Input: part model. Units: mm. Frame: model coordinates. A direction names the side the tool comes from. Round coordinates to 2 decimals unless told otherwise and drop trailing zeros. Order: outer loops, then holes, each group sorted by start corner. A loop starts at its lowest first (then second) coordinate and runs counter-clockwise, first axis right, second up.
Item 1: First-contact query: pin 1 (11 mm diameter, centred on x = 0, z = 5, fed in from -Y). Flat tip, straight axial feed; report the tip coordinate or a pass-through.
Item 2: Cut plane C-C on x = -15. Output: boundary loops of the cut face in (y, z), then the cut area to 3 significant figures.
Item 3: Line query: L1, parallel to X at y = -3.5, z = 6; L2, parallel to Y at x = -16, z = -10.5; L3, parallel to Z at x = -17.5, y = -10.5. Output: solid intervals per line, ascending.
Item 4: Reachability of faces 4 (the flat face through (23, -9, 0)), 5 (the flat face through (-23.4, -15, 11.03)), 6 (the flat face through (0, -9, -11.5)) from +Z, -Z, +X, -X, +Y, -Y: full face, straight path, thin tool, end or side. Return the list, or none.
Item 5: Cut plane A-A on y = -12.75. Output: boundary loops of the cut face in (x, z).
Item 6: Cut plane B-B on z = 1.5. Output: boundary loops of the cut face in (x, y).
Item 7: Cut plane D-D on z = -4.5. Output: boundary loops of the cut face in (x, y).
Item 8: Mould query, pull axis Z, two halves, no side actions, for faces 1 (the flat face through (0, -9, -10.852)), 2 (the flat face through (0, -0.408, 0)), 3 (the cylindrical face through (-18.99, -17.71, -5.81)). Classes: released by +Z, released by -Z, zero draft, split by the parting line, or undercut.
```python
from build123d import *

# Parameters (mm, degrees)
F0_W     = 48
F0_H     = 23
F1_DEPTH = 18
F2_W     = 46
F2_H     = 17
F3_DEPTH = 22.352
F5_DEPTH = 3


with BuildPart() as f1:
    # F0 (on Front) → F1 (new body)
    with BuildSketch(Plane.XZ):
        Rectangle(F0_W, F0_H)
    extrude(amount=F1_DEPTH)

    # F2 (on face) → F3 (cut)
    with BuildSketch(Plane.XY.offset(11.5)):
        with Locations((-4.47e-08, -8.9078345299)):
            Rectangle(F2_W, F2_H)
    extrude(amount=-F3_DEPTH, mode=Mode.SUBTRACT)

    # F4 (on face) → F5 (cut)
    with BuildSketch(Plane.XZ.offset(18)):
        with BuildLine():
            Line((24, 11.5), (-24, 11.5))
            add(Edge.make_bspline(
                [(-24, 11.5), (-21.9359378716, 8.9716693602), (-19.8718757432, 6.4433387205), (-17.8078136148, 4.0833140133)],
                knots=[0, 0, 0, 0, 0.129003883, 0.129003883, 0.129003883, 0.129003883], degree=3))
            ThreePointArc((-17.8078136148, 4.0833140133), (-9.3465218784, 5.5998372929), (-4.6161396554, -1.5776821065))
            ThreePointArc((-4.6161396554, -1.5776821065), (-4.6838516535, -2.6039102527), (-4.8858136092, -3.6123449263))
            ThreePointArc((-4.8858136092, -3.6123449263), (-4.8967692227, -5.2028290958), (-5.482547982, -6.6815525873))
            add(Edge.make_bspline(
                [(-5.482547982, -6.6815525873), (-3.655031988, -7.5874926735), (-1.827515994, -8.0988723785), (0, -8.0988723785)],
                knots=[0.3857802504, 0.3857802504, 0.3857802504, 0.3857802504, 0.5, 0.5, 0.5, 0.5], degree=3))
            add(Edge.make_bspline(
                [(0, -8.0988723785), (1.8266966783, -8.0988723785), (3.6533933566, -7.5879510963), (5.4800900349, -6.6827708081)],
                knots=[0.5, 0.5, 0.5, 0.5, 0.6141685424, 0.6141685424, 0.6141685424, 0.6141685424], degree=3))
            ThreePointArc((5.4800900349, -6.6827708081), (4.8929807707, -5.1976220671), (4.8851620207, -3.6006552741))
            ThreePointArc((4.8851620207, -3.6006552741), (8.4364089916, 5.1373167643), (17.8096110461, 4.085369218))
            add(Edge.make_bspline(
                [(17.8096110461, 4.085369218), (19.8730740307, 6.4448065383), (21.9365370154, 8.9724032691), (24, 11.5)],
                knots=[0.8710335635, 0.8710335635, 0.8710335635, 0.8710335635, 1, 1, 1, 1], degree=3))
        make_face()
        with BuildLine():
            ThreePointArc((-4.6161396554, -1.5776821065), (-9.3465218784, 5.5998372929), (-17.8078136148, 4.0833140133))
            add(Edge.make_bspline(
                [(-17.8078136148, 4.0833140133), (-16.0140889616, 2.0323900412), (-14.2203643085, 0.1085718923), (-12.4266396554, -1.5776821065)],
                knots=[0.129003883, 0.129003883, 0.129003883, 0.129003883, 0.2411116738, 0.2411116738, 0.2411116738, 0.2411116738], degree=3))
            add(Edge.make_bspline(
                [(-12.4266396554, -1.5776821065), (-10.3534160171, -3.5266889647), (-8.2801923789, -5.1583289061), (-6.2069687406, -6.3020449167)],
                knots=[0.2411116738, 0.2411116738, 0.2411116738, 0.2411116738, 0.3706881512, 0.3706881512, 0.3706881512, 0.3706881512], degree=3))
            ThreePointArc((-6.2069687406, -6.3020449167), (-5.4161874116, -5.0211497754), (-4.8858136092, -3.6123449263))
            ThreePointArc((-4.8858136092, -3.6123449263), (-4.6838516535, -2.6039102527), (-4.6161396554, -1.5776821065))
        make_face()
        with BuildLine():
            add(Edge.make_bspline(
                [(-17.8078136148, 4.0833140133), (-16.0140889616, 2.0323900412), (-14.2203643085, 0.1085718923), (-12.4266396554, -1.5776821065)],
                knots=[0.129003883, 0.129003883, 0.129003883, 0.129003883, 0.2411116738, 0.2411116738, 0.2411116738, 0.2411116738], degree=3))
            ThreePointArc((-17.8078136148, 4.0833140133), (-18.9086098616, -5.9352011823), (-9.2157687538, -8.6976693469))
            ThreePointArc((-9.2157687538, -8.6976693469), (-13.0755167796, -6.1542936511), (-12.4266396554, -1.5776821065))
        make_face()
        with BuildLine():
            add(Edge.make_bspline(
                [(-12.4266396554, -1.5776821065), (-10.3534160171, -3.5266889647), (-8.2801923789, -5.1583289061), (-6.2069687406, -6.3020449167)],
                knots=[0.2411116738, 0.2411116738, 0.2411116738, 0.2411116738, 0.3706881512, 0.3706881512, 0.3706881512, 0.3706881512], degree=3))
            ThreePointArc((-12.4266396554, -1.5776821065), (-13.0755167796, -6.1542936511), (-9.2157687538, -8.6976693469))
            ThreePointArc((-9.2157687538, -8.6976693469), (-7.5616079145, -7.6879502193), (-6.2069687406, -6.3020449167))
        make_face()
        with BuildLine():
            ThreePointArc((-6.2069687406, -6.3020449167), (-7.5616079145, -7.6879502193), (-9.2157687538, -8.6976693469))
            ThreePointArc((-9.2157687538, -8.6976693469), (-7.0845998748, -8.1794909589), (-5.482547982, -6.6815525873))
            add(Edge.make_bspline(
                [(-6.2069687406, -6.3020449167), (-5.9654951544, -6.4352564051), (-5.7240215682, -6.5618487914), (-5.482547982, -6.6815525873)],
                knots=[0.3706881512, 0.3706881512, 0.3706881512, 0.3706881512, 0.3857802504, 0.3857802504, 0.3857802504, 0.3857802504], degree=3))
        make_face()
        with BuildLine():
            ThreePointArc((20.2391303397, -1.5758105962), (19.606097165, 1.5044296902), (17.8096110461, 4.085369218))
            add(Edge.make_bspline(
                [(12.4286303397, -1.5758105962), (14.2222905752, 0.1105585898), (16.0159508106, 2.0344340033), (17.8096110461, 4.085369218)],
                knots=[0.7589297987, 0.7589297987, 0.7589297987, 0.7589297987, 0.8710335635, 0.8710335635, 0.8710335635, 0.8710335635], degree=3))
            ThreePointArc((12.4286303397, -1.5758105962), (13.080424676, -6.1500390798), (9.2274737476, -8.7001706883))
            ThreePointArc((9.2274737476, -8.7001706883), (16.6713462557, -8.1334985962), (20.2391303397, -1.5758105962))
        make_face()
        with BuildLine():
            add(Edge.make_bspline(
                [(12.4286303397, -1.5758105962), (14.2222905752, 0.1105585898), (16.0159508106, 2.0344340033), (17.8096110461, 4.085369218)],
                knots=[0.7589297987, 0.7589297987, 0.7589297987, 0.7589297987, 0.8710335635, 0.8710335635, 0.8710335635, 0.8710335635], degree=3))
            ThreePointArc((17.8096110461, 4.085369218), (8.4364089916, 5.1373167643), (4.8851620207, -3.6006552741))
            ThreePointArc((4.8851620207, -3.6006552741), (5.4160889034, -5.0150216763), (6.2093732837, -6.300718206))
            add(Edge.make_bspline(
                [(6.2093732837, -6.300718206), (8.282458969, -5.1567010835), (10.3555446544, -3.5248908904), (12.4286303397, -1.5758105962)],
                knots=[0.6293619434, 0.6293619434, 0.6293619434, 0.6293619434, 0.7589297987, 0.7589297987, 0.7589297987, 0.7589297987], degree=3))
        make_face()
        with BuildLine():
            ThreePointArc((-4.8858136092, -3.6123449263), (-5.4161874116, -5.0211497754), (-6.2069687406, -6.3020449167))
            add(Edge.make_bspline(
                [(-6.2069687406, -6.3020449167), (-5.9654951544, -6.4352564051), (-5.7240215682, -6.5618487914), (-5.482547982, -6.6815525873)],
                knots=[0.3706881512, 0.3706881512, 0.3706881512, 0.3706881512, 0.3857802504, 0.3857802504, 0.3857802504, 0.3857802504], degree=3))
            ThreePointArc((-5.482547982, -6.6815525873), (-4.8967692227, -5.2028290958), (-4.8858136092, -3.6123449263))
        make_face()
        with BuildLine():
            ThreePointArc((9.2274737476, -8.7001706883), (13.080424676, -6.1500390798), (12.4286303397, -1.5758105962))
            add(Edge.make_bspline(
                [(6.2093732837, -6.300718206), (8.282458969, -5.1567010835), (10.3555446544, -3.5248908904), (12.4286303397, -1.5758105962)],
                knots=[0.6293619434, 0.6293619434, 0.6293619434, 0.6293619434, 0.7589297987, 0.7589297987, 0.7589297987, 0.7589297987], degree=3))
            ThreePointArc((6.2093732837, -6.300718206), (7.5680345553, -7.6896080143), (9.2274737476, -8.7001706883))
        make_face()
        with BuildLine():
            ThreePointArc((6.2093732837, -6.300718206), (5.4160889034, -5.0150216763), (4.8851620207, -3.6006552741))
            ThreePointArc((4.8851620207, -3.6006552741), (4.8929807707, -5.1976220671), (5.4800900349, -6.6827708081))
            add(Edge.make_bspline(
                [(5.4800900349, -6.6827708081), (5.7231844512, -6.5623105935), (5.9662788674, -6.4348680757), (6.2093732837, -6.300718206)],
                knots=[0.6141685424, 0.6141685424, 0.6141685424, 0.6141685424, 0.6293619434, 0.6293619434, 0.6293619434, 0.6293619434], degree=3))
        make_face()
        with BuildLine():
            ThreePointArc((9.2274737476, -8.7001706883), (7.5680345553, -7.6896080143), (6.2093732837, -6.300718206))
            add(Edge.make_bspline(
                [(5.4800900349, -6.6827708081), (5.7231844512, -6.5623105935), (5.9662788674, -6.4348680757), (6.2093732837, -6.300718206)],
                knots=[0.6141685424, 0.6141685424, 0.6141685424, 0.6141685424, 0.6293619434, 0.6293619434, 0.6293619434, 0.6293619434], degree=3))
            ThreePointArc((5.4800900349, -6.6827708081), (7.0883105329, -8.1845921438), (9.2274737476, -8.7001706883))
        make_face()
    extrude(amount=-F5_DEPTH, mode=Mode.SUBTRACT)


solid = f1.part
```
From the geometry:
1. pin 1: stops at y = -0.41
2. outline: (-18, -11.5) - (0, -11.5) - (0, 11.5) - (-0.41, 11.5) - (-0.41, -10.85) - (-17.41, -10.85) - (-17.41, -8.95) - (-18, -8.95) - close
2. area: 21.9 mm2
3. L1: x = -24 to -23, 23 to 24
3. L2: y = -18 to -17.41, -0.41 to 0
3. L3: z = -11.5 to -10.85
4. face 4: +Z
4. face 5: +Z, -Y
4. face 6: -Z, +X, -X, +Y, -Y
5. outline: (-24, -11.5) - (24, -11.5) - (24, 11.5) - (23, 11.5) - (23, -10.85) - (-23, -10.85) - (-23, 11.5) - (-24, 11.5) - close
6. outline: (-24, -18) - (-19.61, -18) - (-19.61, -17.41) - (-23, -17.41) - (-23, -0.41) - (23, -0.41) - (23, -17.41) - (19.61, -17.41) - (19.61, -18) - (24, -18) - (24, 0) - (-24, 0) - close
7. outline: (-24, -18) - (-19.67, -18) - (-19.67, -17.41) - (-23, -17.41) - (-23, -0.41) - (23, -0.41) - (23, -17.41) - (19.67, -17.41) - (19.67, -18) - (24, -18) - (24, 0) - (-24, 0) - close
8. face 1: released by +Z
8. face 2: zero draft
8. face 3: undercut
